Study the drawing (mm; zero at the part's minimum x, y, z) and answer. Coordinates: 2 decimals unless noted, no trailing zeros. Write each loop counter-clockwise with the first axis right and the second up, starting at its lowest first coordinate (ties: lowest second). Pieces come first, ordered by that corner, then holes. Notation, with made-up numbers: (-32.5, 2) -> (-3.5, 2) arc R19 ccw to (-3.5, 33) -> close; hole circle Ø10 at (71, 74). An arc over 180 degrees is marked (long way). Write item = value, one per line. Start each with the question number.
1) For a pull along Y with two mould halves and no side action, classify the marked faces 1, 2 and 3 as released by +Y, released by -Y, zero draft, split by the parting line, or undercut.
2) Section D-D (y = 5.5) is taken. Determine the outline of the cut face in (x, z).
3) Flat-ended cylindrical pins translate along their axes: pin 1 Ø3 at (y, z) = (4.5, 9.5) entering from -X; pin 2 Ø3 at (x, z) = (0.5, 3) entering from -Y; pin 3 Ø3 at (y, z) = (4, 9) entering from +X; pin 4 Ø1.1 at (x, y) = (0.5, 3.5) entering from +Z. Find the tip coordinate at first contact, or state that the pin passes through.
4) Find the intervals of material crossed by line 1 along Z through (x, y) = (3, 4); line 2 along X through (y, z) = (5.75, 10.5); line 3 along Y through (x, z) = (1.9, 10.5), in increasing order. Write a range as from..to.
5) Section C-C (x = 2.3) is taken. Determine the outline of the cut face in (y, z).
6) Section B-B (y = 4) is taken. Determine the outline of the cut face in (x, z), plus the area to 3 significant figures.
7) Section A-A (z = 9) is taken. Determine the outline of the cut face in (x, y), plus the area to 3 significant figures.
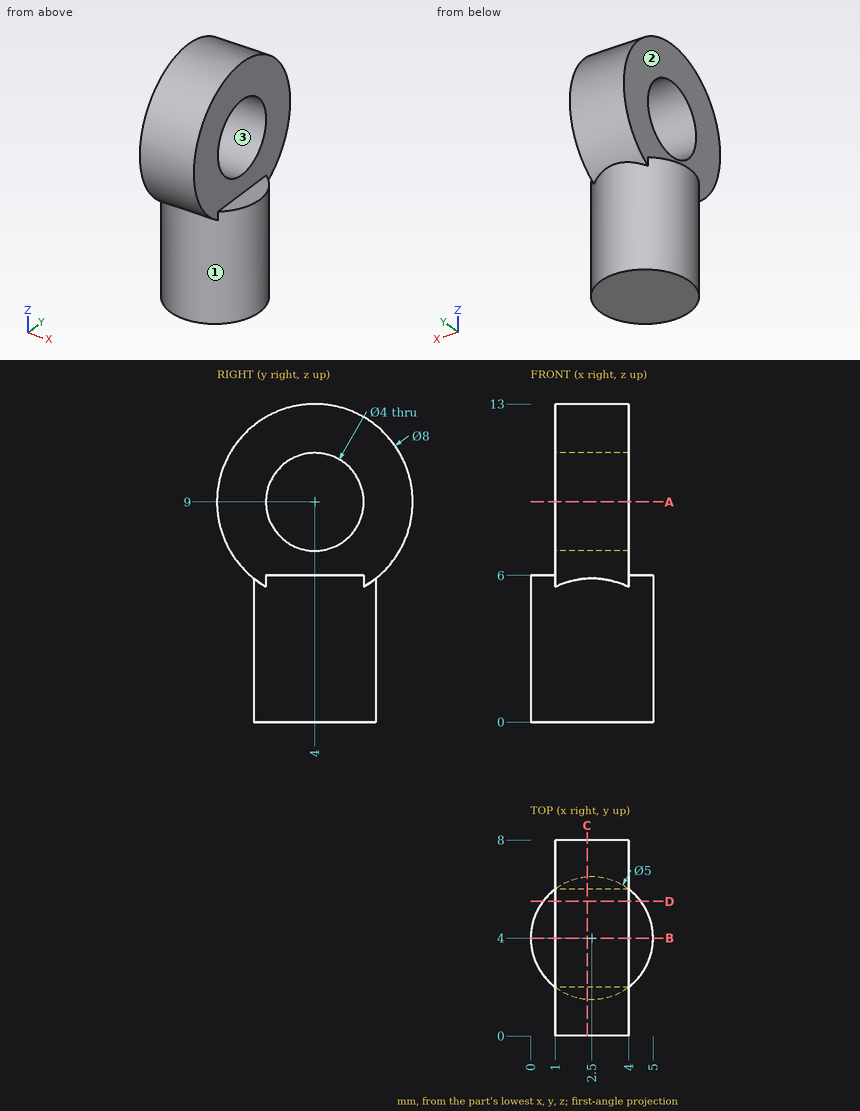
Answer key:
q1.face_1 = split by the parting line
q1.face_2 = zero draft
q1.face_3 = undercut
q2.outline = (0.5, 0) -> (4.5, 0) -> (4.5, 6) -> (4, 6) -> (4, 7.68) -> (1, 7.68) -> (1, 6) -> (0.5, 6) -> close; (1, 10.32) -> (4, 10.32) -> (4, 12.71) -> (1, 12.71) -> close
q3.pin_1 = 1
q3.pin_2 = 1.55
q3.pin_3 = through
q3.pin_4 = 12.99
q4.line_1 = 0..7, 11..13
q4.line_2 = 1..4
q4.line_3 = 0.29..2.68, 5.32..7.71
q5.outline = (1.51, 0) -> (6.49, 0) -> (6.49, 5.87) arc R4 ccw (long way) to (1.51, 5.87) -> close; hole circle Ø4 at (4, 9)
q6.outline = (0, 0) -> (5, 0) -> (5, 6) -> (4, 6) -> (4, 7) -> (1, 7) -> (1, 6) -> (0, 6) -> close; (1, 11) -> (4, 11) -> (4, 13) -> (1, 13) -> close
q6.area = 39.0 mm^2
q7.outline = (1, 0) -> (4, 0) -> (4, 2) -> (1, 2) -> close; (1, 6) -> (4, 6) -> (4, 8) -> (1, 8) -> close
q7.area = 12.0 mm^2
